Design review of the part shown in the three views and the two pictorial views. Dimensions are in mm from the part's minimum x, y and z. A direction names the side the tool comes from. Give positions to 0.01 mm unless a question says otherwise; leave off trailing zeros. Write each loop counter-clockwise with the first axis right and the second up, starting at its lowest first coordinate (ties: lowest second). Pieces come first, ordered by that corner, then holes. Notation, with made-up numbers: (-28, -4.75) -> (-6, -4.75) arc R34 cw to (-6, 29.25) -> close; hole circle Ø4 at (-39.5, 18). An arc over 180 degrees is marked (long way). Use CSV: the item, a comma, the result in double quotes.
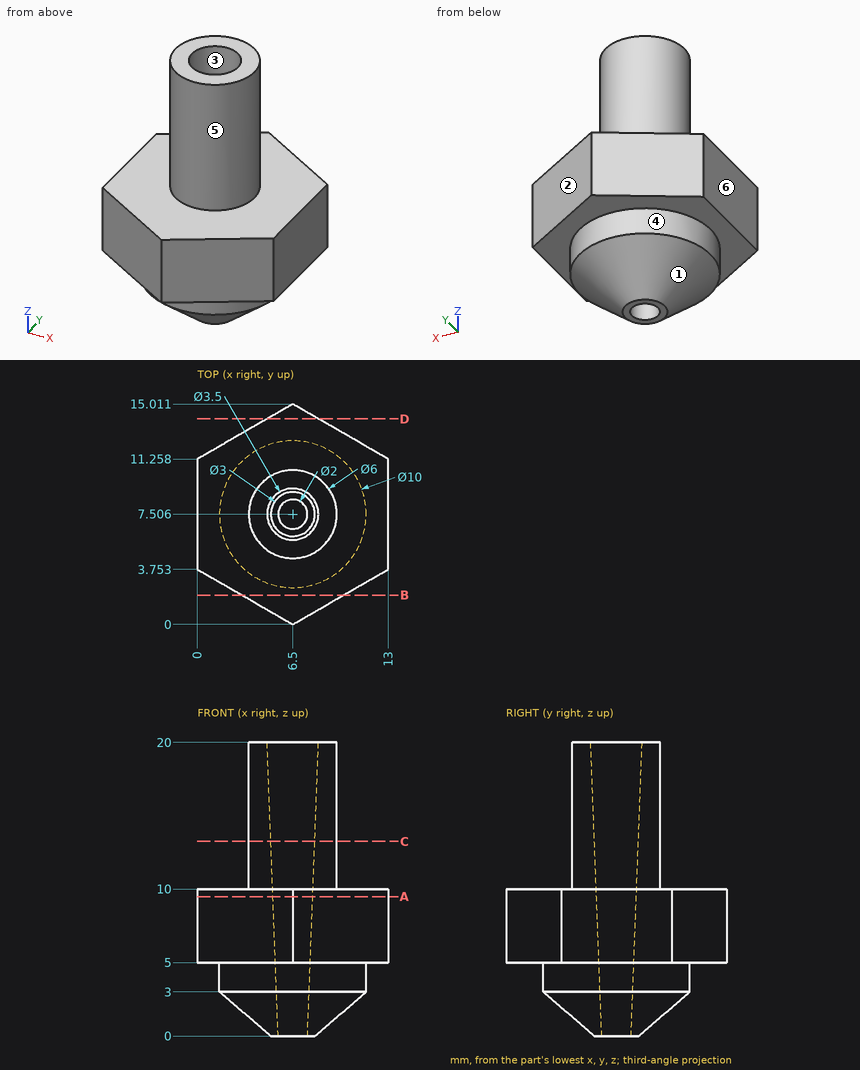
Q1. To check wall thickness, follow probe 1 along X at (y, z) = (7.5, 10.25) (1 decimal); probe 2 along Y at (x, z) = (5.25, 10.25) (1 decimal); probe 3 along Z at (x, y) = (1.75, 9.25). State the ranges of each line that lie inside material, in increasing order.
Derived:
probe 1,"x = 3.5 to 5.1, 7.9 to 9.5"
probe 2,"y = 4.8 to 6.9, 8.1 to 10.2"
probe 3,"z = 5 to 10"
Q2. Consider section D-D (y = 14). Write out the cut boundary in (x, z).
Derived:
outline,"(4.75, 5) -> (8.25, 5) -> (8.25, 10) -> (4.75, 10) -> close"
Q3. Machinability: for the marked faces 4, 5 and 6, which of the approach directions +Z, -Z, +X, -X, +Y, -Y give a long, thin tool a straight path to every point of the face, cutting with its end or side? Answer none if there is none.
Derived:
face 4,"-Z"
face 5,"+Z"
face 6,"+Z, -Z, -X, +Y, -Y"
Q4. Insertion check: pin 1 (1 mm diameter, centred on x = 1.5, y = 6, fed in from +Z); pin 2 (2 mm diameter, centred on y = 6.5, z = 18, fed in from -X); pin 3 (1 mm diameter, centred on x = 5, y = 3.5, fed in from -Z). Each pin has a flat end and moves straight along its axis. Give the tip position at first contact, or say it passes through.
Derived:
pin 1,"stops at z = 10"
pin 2,"stops at x = 3.5"
pin 3,"stops at z = 1.95"
Q5. Consider section A-A (z = 9.5). Write out the cut boundary in (x, y) (1 decimal).
Derived:
outline,"(0, 3.8) -> (6.5, 0) -> (13, 3.8) -> (13, 11.3) -> (6.5, 15) -> (0, 11.3) -> close; hole circle Ø2.7 at (6.5, 7.5)"
Q6. The part is to be moulded in two halves that separate along Y. For the marked faces 1, 2 and 3, say which applies: pulls with the +Y half, pulls with the -Y half, needs draft (parallel to the pull), parting line crosses it, or undercut.
Derived:
face 1,"parting line crosses it"
face 2,"pulls with the +Y half"
face 3,"undercut"
Q7. Consider section B-B (y = 2). Write out the cut boundary in (x, z) (1 decimal).
Derived:
outline,"(3, 5) -> (10, 5) -> (10, 10) -> (3, 10) -> close"
Q8. Consider section C-C (z = 13.25). Write out the cut boundary in (x, y) (1 decimal).
Derived:
outline,"circle Ø6 at (6.5, 7.5); hole circle Ø3 at (6.5, 7.5)"
